Job drawing, mm, ordinate dimensions from the low corner. One solid piece. Give positions to 0.01 mm unless a question says otherwise; leave off trailing zeros. Loops run counter-clockwise (first coordinate to the right, second up) from the corner with the lowest first, then second, coordinate; pieces in that order, holes last.
Item 1: Saw through at C-C on x = 20.5. Give the cut face in (y, z) (1 decimal).
Item 2: Drop flat-ended pins along their axis: P1, Ø5.5, axis at x = 20.5, z = 9.89, coming from the -Y side; P2, Ø3, axis at x = 11.5, y = 7.5, coming from the +Z side; P3, Ø4, axis at y = 8, z = 15, coming from the +X side; P4, Ø4, axis at x = 20.5, z = 60.11, coming from the +Y side. Give the stop position or say it passes through.
Item 3: Mould opens along X. For the marked faces 1, 2 and 3 say: released by +X, released by -X, zero draft, split by the parting line, or undercut.
Item 4: Probe probe 1 along Z at (x, y) = (20.5, 12) (1 decimal); probe 2 along X at (y, z) = (1.7, 35); probe 3 along X at (y, z) = (8.75, 24.5). List the from-to ranges inside material, lowest first.
Item 5: Saw through at B-B on z = 35. Give the cut face in (x, y).
Item 6: Saw through at D-D on y = 9.5. Give the number of separate pieces and of enclosed holes in the cut face, plus the area to 3 significant figures.
Item 7: Saw through at A-A on x = 35. Give the cut face in (y, z).
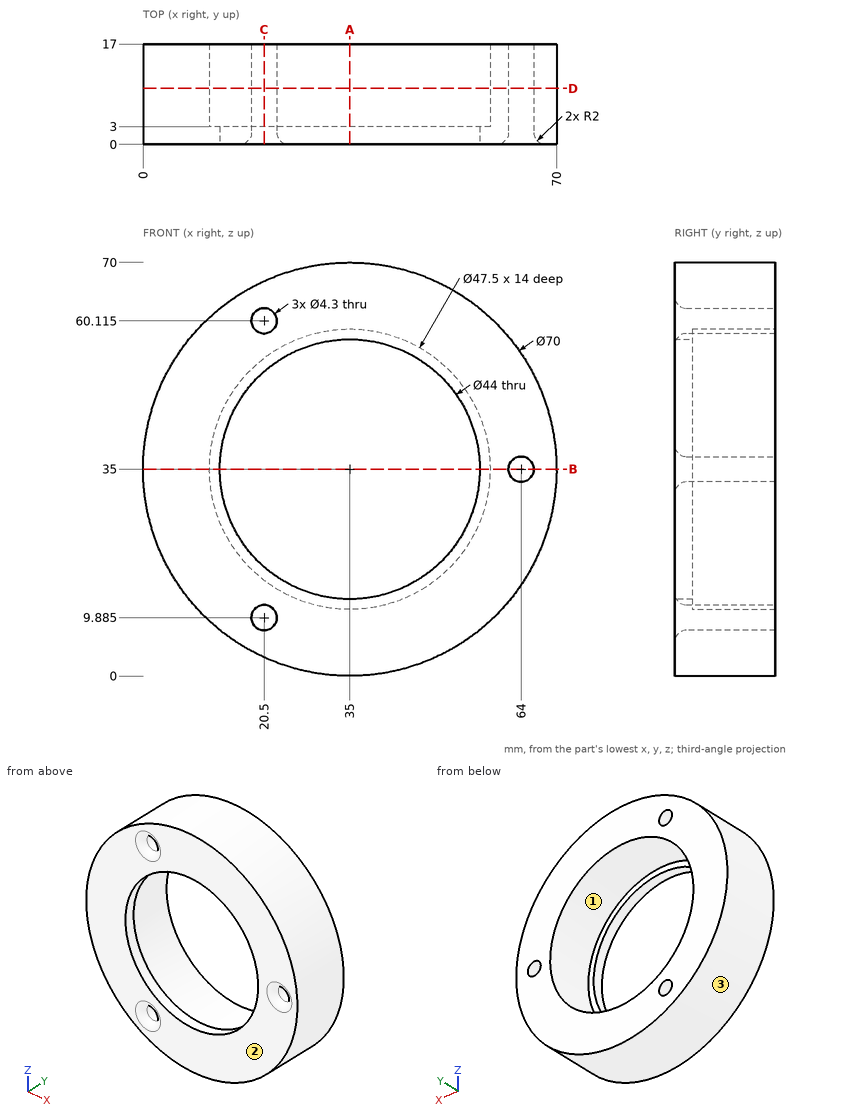
Results below:
1. outline: (0, 3.1) - (17, 3.1) - (17, 7.7) - (2, 7.7) arc R2 ccw to (0, 5.7) - close; (0, 14) arc R2 ccw to (2, 12) - (17, 12) - (17, 16.2) - (3, 16.2) - (3, 18.5) - (0, 18.5) - close; (0, 51.5) - (3, 51.5) - (3, 53.8) - (17, 53.8) - (17, 58) - (2, 58) arc R2 ccw to (0, 56) - close; (0, 64.3) arc R2 ccw to (2, 62.3) - (17, 62.3) - (17, 66.9) - (0, 66.9) - close
2. P1: stops at y = 0.57
2. P2: stops at z = 62.22
2. P3: stops at x = 65.02
2. P4: passes through
3. face 1: undercut
3. face 2: zero draft
3. face 3: split by the parting line
4. probe 1: z = 3.1 to 7.7, 12 to 16.2, 53.8 to 58, 62.3 to 66.9
4. probe 2: x = 0 to 13, 57 to 61.83, 66.17 to 70
4. probe 3: x = 1.61 to 13.7, 56.3 to 68.39
5. outline: (0, 0) - (13, 0) - (13, 3) - (11.25, 3) - (11.25, 17) - (0, 17) - close; (57, 0) - (59.85, 0) arc R2 ccw to (61.85, 2) - (61.85, 17) - (58.75, 17) - (58.75, 3) - (57, 3) - close; (66.15, 2) arc R2 ccw to (68.15, 0) - (70, 0) - (70, 17) - (66.15, 17) - close
6. separate pieces: 1
6. enclosed holes: 4
6. area: 2,030 mm2
7. outline: (0, 0) - (17, 0) - (17, 11.25) - (3, 11.25) - (3, 13) - (0, 13) - close; (0, 57) - (3, 57) - (3, 58.75) - (17, 58.75) - (17, 70) - (0, 70) - close
